Geometry check sheet. Reference: the model listing, model coordinates, mm. Round coordinates to 2 decimals unless told otherwise and drop trailing zeros. Order: outer loops, then holes, each group sorted by start corner. A loop starts at its lowest first (then second) coordinate and runs counter-clockwise, first axis right, second up. Notation, with made-up numbers: (3.25, -27.5) -> (35.25, -27.5) arc R32 cw to (35.25, 6.5) -> close; hole circle Ø8 at (-32, -39). An arc over 180 degrees is marked (long way). Use a Markdown table: item, result. Add a question column.
Item 1: Sectioned sample at B-B, the plane x = -0.5. Record the cut outline in (y, z), and give its area (3 significant figures).
Item 2: Sectioned sample at A-A, the plane y = 1.05. Record the cut outline in (x, z).
Item 3: Gauge pin test, flat ends, axial feed: pin 1 Ø1.5 at (x, y) = (-8.5, 2) entering from +Z; pin 2 Ø1.5 at (y, z) = (1, 2) entering from -X; pin 3 Ø3 at (y, z) = (1.5, 4) entering from +X. Record the tip position at first contact, or that the pin passes through.
Item 4: Sectioned sample at C-C, the plane z = -5. Record the cut outline in (x, y).
Item 5: Material ranges on probe 1 along X at (y, z) = (2.95, 0); probe 2 along Z at (x, y) = (-52.5, 4.4); probe 3 along Z at (x, y) = (-27, 1.05), recorded low to high. Write a range as [from, to].
Item 6: Mould release check, pull along Z, two halves, no side actions. Record for faces 1 (the flat face through (-4, 5, 0)), 2 (the cylindrical face through (45.78, 2.46, -0.07)), 3 (the cylindrical face through (-67.44, 2.46, 0.24)): pulls with the +Z half, pulls with the -Z half, needs draft (parallel to the pull), parting line crosses it, or undercut.
from build123d import *

# Parameters (mm, degrees)
SKETCH1_R               = 1.05
SKETCH1_R_2             = 1.5
BOSS_EXTRUDE1_DEPTH     = 5
SKETCH2_R               = 1
CUT_EXTRUDE1_DEPTH      = 1
CUT_EXTRUDE1_DEPTH_BACK = 6


with BuildPart() as part:
    # Sketch1 → Boss-Extrude1 (new body)
    with BuildSketch(Plane(origin=(0, 0, 0), x_dir=(1, 0, 0), z_dir=(0, 1, 0))):
        with BuildLine():
            Line((-50.348842759, 14.527458054), (47.631245247, 10.594116014))
            ThreePointArc((47.631245247, 10.594116014), (57.878041754, 0.037488485), (47.706171294, -10.591353165))
            Line((47.706171294, -10.591353165), (-50.583585242, -14.563860903))
            ThreePointArc((-50.583585242, -14.563860903), (-67.441412758, 0.118774156), (-50.348842759, 14.527458054))
        make_face()
        with Locations((-52.721891954, 0)):
            Circle(SKETCH1_R, mode=Mode.SUBTRACT)
        with Locations((47.278108046, 0)):
            Circle(SKETCH1_R_2, mode=Mode.SUBTRACT)
    extrude(amount=BOSS_EXTRUDE1_DEPTH)

    # Sketch2 → Cut-Extrude1 (cut, two sides)
    with BuildSketch(Plane(origin=(0, 5, 0), x_dir=(1, 0, 0), z_dir=(0, 1, 0))) as cut_extrude1_sk:
        with Locations((-38.271891954, 0)):
            Circle(SKETCH2_R)
    extrude(amount=CUT_EXTRUDE1_DEPTH, mode=Mode.SUBTRACT)
    extrude(cut_extrude1_sk.sketch, amount=-CUT_EXTRUDE1_DEPTH_BACK, mode=Mode.SUBTRACT)


solid = part.part
Found:
| question | item | result |
|---|---|---|
| 1 | outline | (0, -12.53) -> (5, -12.53) -> (5, 12.54) -> (0, 12.54) -> close |
| 1 | area | 125 mm2 |
| 2 | outline | (-50.58, 14.56) arc R14.72 ccw (long way) to (-50.35, -14.53) -> (47.63, -10.59) arc R10.6 ccw to (47.71, 10.59) -> close; hole circle Ø2.1 at (-52.72, 0); hole circle Ø2 at (-38.27, 0); hole circle Ø3 at (47.28, 0) |
| 3 | pin 1 | stops at z = 12.89 |
| 3 | pin 2 | stops at x = -67.39 |
| 3 | pin 3 | stops at x = 57.58 |
| 4 | outline | (-66.57, 0) -> (56.62, 0) -> (56.62, 5) -> (-66.57, 5) -> close |
| 5 | probe 1 | x = [-67.44, -53.77], [-51.67, -39.27], [-37.27, 45.78], [48.78, 57.88] |
| 5 | probe 2 | z = [-14.72, -1.03], [1.03, 14.72] |
| 5 | probe 3 | z = [-13.59, 13.61] |
| 6 | face 1 | needs draft |
| 6 | face 2 | undercut |
| 6 | face 3 | parting line crosses it |
